Read the model definition and answer for the solid it produces. Units are mm, in the model's axes. A direction names the side the tool comes from. Coordinates: 2 decimals unless noted, no trailing zeros. Loops run counter-clockwise (first coordinate to the right, second up) from the corner with the lowest first, then second, coordinate; pieces in that order, holes last. Notation, with made-up numbers: M 32,34.25 L 36,34.25 A16 cw 36,38.25 Z; hole C 43,-19 d1. An arc over 180 degrees is marked long. Put each result on its own line as item: value.
from build123d import *

# Parameters (mm, degrees)
BOSS_EXTRUDE1_DEPTH                             = 4.7625
CBORE_FOR_10_BUTTON_HEAD_CAP_SCREW1_D           = 4.9784
CBORE_FOR_10_BUTTON_HEAD_CAP_SCREW1_CBORE_D     = 9.92124
CBORE_FOR_10_BUTTON_HEAD_CAP_SCREW1_CBORE_DEPTH = 2.5654


with BuildPart() as part:
    # Sketch1 → Boss-Extrude1 (new body)
    with BuildSketch(Plane(origin=(0, 0, 0), x_dir=(1, 0, 0), z_dir=(0, 1, 0))):
        with BuildLine():
            Line((40, -50), (-40, -50))
            ThreePointArc((-40, -50), (-54.142135624, -44.142135624), (-60, -30))
            Line((-60, -30), (-60, 30))
            ThreePointArc((-60, 30), (-54.142135624, 44.142135624), (-40, 50))
            Line((-40, 50), (40, 50))
            ThreePointArc((40, 50), (54.142135624, 44.142135624), (60, 30))
            Line((60, 30), (60, -30))
            ThreePointArc((60, -30), (54.142135624, -44.142135624), (40, -50))
        make_face()
    extrude(amount=BOSS_EXTRUDE1_DEPTH)

    # CBORE for #10 Button Head Cap Screw1 (through all)
    with Locations(Plane(origin=(0, 4.7625, 0), x_dir=(1, 0, 0), z_dir=(0, 1, 0))):
        with Locations((29.185832393, 29.185832393), (29.185832393, -29.185832393), (-29.185832393, -29.185832393), (-29.185832393, 29.185832393)):
            CounterBoreHole(CBORE_FOR_10_BUTTON_HEAD_CAP_SCREW1_D / 2, CBORE_FOR_10_BUTTON_HEAD_CAP_SCREW1_CBORE_D / 2, CBORE_FOR_10_BUTTON_HEAD_CAP_SCREW1_CBORE_DEPTH)


solid = part.part
1) Which of the six approach directions +Z, -Z, +X, -X, +Y, -Y give full straight-line access (tool end or side, diameter ignored) to faces 1 (the flat face through (-27, 2.197, 31)), 2 (the flat face through (-1, 2, -50))?
Answer list:
face 1: +Y
face 2: -Z, +X, -X, +Y, -Y
2) Find section B-B, the plane y = 1.3. Write down the section's boundary in (x, z).
Answer list:
outline: M -60,-30 A20 ccw -40,-50 L 40,-50 A20 ccw 60,-30 L 60,30 A20 ccw 40,50 L -40,50 A20 ccw -60,30 Z; hole C -29.19,-29.19 d4.98; hole C -29.19,29.19 d4.98; hole C 29.19,-29.19 d4.98; hole C 29.19,29.19 d4.98
3) Find section D-D, the plane z = 38. Write down the section's boundary in (x, y), plus the area to 3 significant figures.
Answer list:
outline: M -58.33,0 L 58.33,0 L 58.33,4.76 L -58.33,4.76 Z
area: 556 mm^2
4) Find section A-A, the plane x = 30. Write down the section's boundary in (y, z).
Answer list:
outline: M 0,-50 L 4.76,-50 L 4.76,-34.08 L 2.2,-34.08 L 2.2,-31.54 L 0,-31.54 Z; M 0,-26.83 L 2.2,-26.83 L 2.2,-24.29 L 4.76,-24.29 L 4.76,24.29 L 2.2,24.29 L 2.2,26.83 L 0,26.83 Z; M 0,31.54 L 2.2,31.54 L 2.2,34.08 L 4.76,34.08 L 4.76,50 L 0,50 Z
5) Given pin 1 Ø8 at (x, z) = (29.19, -29.19) entering from +Y; pin 2 Ø4.5 at (x, z) = (-29.19, -29.19) entering from -Y, each flat-ended and moving along its own axis, determine where each tip first touches the part or whether it passes through.
Answer list:
pin 1: stops at y = 2.2
pin 2: passes through
6) Find section C-C, the plane x = -28.5. Write down the section's boundary in (y, z), plus the area to 3 significant figures.
Answer list:
outline: M 0,-50 L 4.76,-50 L 4.76,-34.1 L 2.2,-34.1 L 2.2,-31.58 L 0,-31.58 Z; M 0,-26.79 L 2.2,-26.79 L 2.2,-24.27 L 4.76,-24.27 L 4.76,24.27 L 2.2,24.27 L 2.2,26.79 L 0,26.79 Z; M 0,31.58 L 2.2,31.58 L 2.2,34.1 L 4.76,34.1 L 4.76,50 L 0,50 Z
area: 405 mm^2
7) Straight lines are drawn through the part: line 1 (X direction, y = 3.05, z = 29.5); line 2 (X direction, y = 3.5, z = -30); line 3 (Z direction, x = 27.5, y = 4.1). For each, find the intervals that lie inside material, in ascending order. Write a range as [from, to].
Answer list:
line 1: x = [-60, -34.14], [-24.24, 24.24], [34.14, 60]
line 2: x = [-60, -34.08], [-24.29, 24.29], [34.08, 60]
line 3: z = [-50, -33.85], [-24.52, 24.52], [33.85, 50]
8) Determine the mould class of faces 3 (the flat face through (60, 2, 0)), 4 (the cylindrical face through (-24.603, 3.498, 31.086)), 5 (the flat face through (1, 4.762, -1)) for opening direction X: released by +X, released by -X, zero draft, split by the parting line, or undercut.
Answer list:
face 3: released by +X
face 4: undercut
face 5: zero draft
